Geometry: final body of the model. Coordinates: model frame, mm. A direction names the side the tool comes from. Coordinates: 2 decimals unless noted, no trailing zeros. Loops run counter-clockwise (first coordinate to the right, second up) from the corner with the lowest first, then second, coordinate; pieces in that order, holes last. Notation, with made-up numbers: (28.5, -1) -> (58.5, -1) arc R11 cw to (58.5, 3) -> close; hole circle Ø7 at (64, -8). An arc over 180 degrees is marked (long way). One line per item, written item: value. Start each with the question number.
Item 1: Set-up query: faces 4 (the cylindrical face through (-3.958, 1.986, 33.505)), 5 (the cylindrical face through (-1.203, 1.768, 60.988)). Return all of +Z, -Z, +X, -X, +Y, -Y with unobstructed straight access to the full face (end or side cutting, diameter ignored); none if empty.
Item 2: Mould query, pull axis X, two halves, no side actions, for faces 1 (the flat face through (-49, 2, 62.128)), 2 (the cylindrical face through (-96.47, 1.77, 60.93)), 3 (the flat face through (-4, 1, 31)). Classes: +X half, -X half, draft (parallel to the pull), parting line (faces both ways), or undercut.
Item 3: Section query A-A on z = 2. Return loops of the section in (x, y).
Item 4: Contact query for a flat-ended pin moving along its axis: pin 1 Ø3 at (x, z) = (-4.5, 31.06) entering from +Y. Output: stop coordinate, or through.
Item 5: Ray query, probe 1 along X at (y, z) = (1.55, 2); probe 2 along Z at (x, y) = (-5, 1.65). Return the intervals inside material, ascending. Write a range as from..to.
Autodesk Inventor part; units mm, degrees
ref_plane "YZ Plane" through (0, 0, 0) normal (1, 0, 0) x (0, 1, 0)
ref_plane "XZ Plane" through (0, 0, 0) normal (0, 1, 0) x (-1, 0, 0)
ref_plane "XY Plane" through (0, 0, 0) normal (0, 0, 1) x (1, 0, 0)
sketch "Sketch1" plane through (0, 0, 0) normal (0, 1, 0) x (-1, 0, 0)
  line L0 (0, 0) -> (97.6122, 0)
  line L1 (97.6122, 0) -> (97.6122, 62.1284)
  line L2 (97.6122, 62.1284) -> (0, 62.1284)
  line L3 (0, 62.1284) -> (0, 0)
  line L4 (97.6122, 62.1284) -> (97.6122, 60.1284)
  line L5 (97.6122, 60.1284) -> (74.5998, 60.1284)
  circle A0 centre (74.5998, 60.1284) radius 1
  line L6 (0, 31.0642) -> (4.5, 31.0642)
  circle A1 centre (4.5, 31.0642) radius 2.5
  line L7 (4.5, 31.0642) -> (97.6122, 31.0642)
  circle A2 centre (74.5998, 2) radius 1
  dimension "d0" = 97.6122
  dimension "d1" = 62.1284
  dimension "d2" = 2
  dimension "d3" = 23.0124
  dimension "d4" = 2
  dimension "d5" = 4.5
  dimension "d6" = 5
extrude "Extrusion1" add sketch "Sketch1" along normal blind 3 contours L3 L6 A1 L7 L1 L0 | L3 L2 L1 L7 A1 L6
extrude "Extrusion2" add sketch "Sketch1" along normal blind 1 contours A1 L7 L6 | L6 L7 A1 | A0 | A2
fillet "Fillet1" radius 4 4 edges at (-97.6122, 1.5, 62.1284) (-97.6122, 1.5, 0) (0, 1.5, 0) (0, 1.5, 62.1284)
move faces "Move1" translate (0, 0.5, 0) faces at (-63.7415, 0, 20.7095)
properties part number "magnet card top"
Reply:
1. face 4: +Y
1. face 5: +Z, +X, +Y, -Y
2. face 1: draft
2. face 2: -X half
2. face 3: undercut
3. outline: (-97.08, 0.5) -> (-0.54, 0.5) -> (-0.54, 3) -> (-73.6, 3) -> (-73.6, 1) -> (-75.6, 1) -> (-75.6, 3) -> (-97.08, 3) -> close
4. pin 1: stops at y = 1
5. probe 1: x = -97.08..-75.6, -73.6..-0.54
5. probe 2: z = 0..28.61, 33.51..62.13
